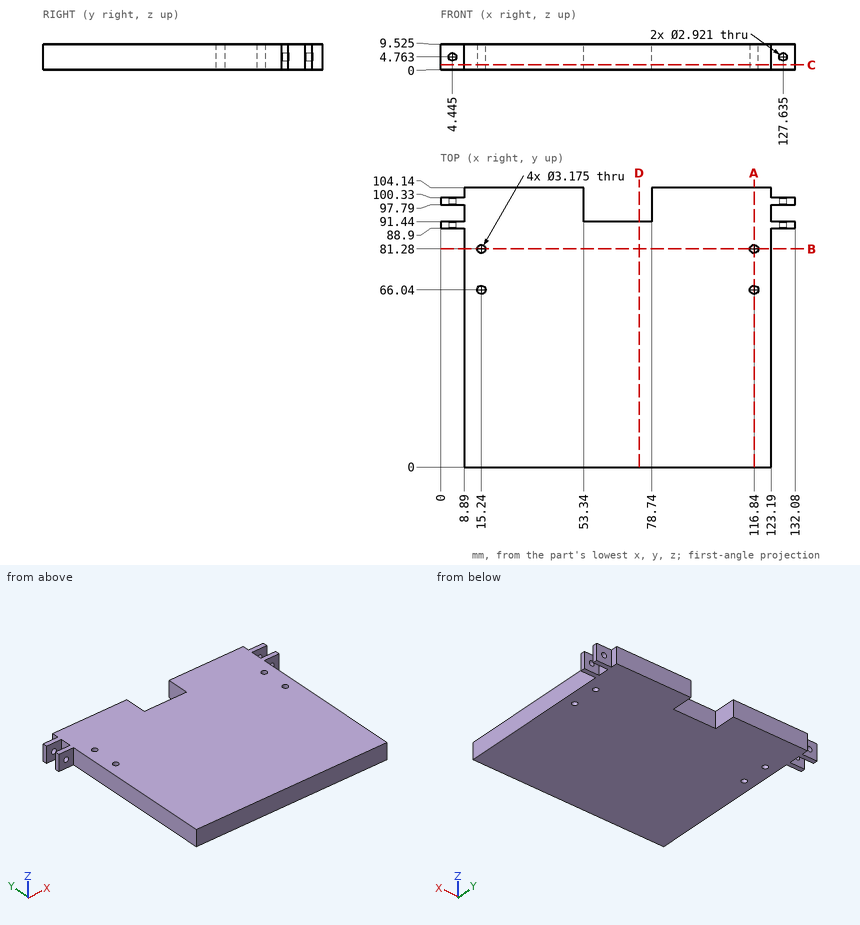
Design review of the part shown in the three views and the two pictorial views. Dimensions are in mm from the part's minimum x, y and z. Round coordinates to 2 decimals unless told otherwise and drop trailing zeros. Write each loop counter-clockwise with the first axis right and the second up, starting at its lowest first coordinate (ties: lowest second). Pieces come first, ordered by that corner, then holes. Notation, with made-up numbers: (-25.75, 83.25) - (32.25, 83.25) arc R20 ccw to (32.25, 94.25) - close; hole circle Ø3 at (63, 46.25). An arc over 180 degrees is marked (long way). Answer as CSV lines item,"result". Start each with the question number.
(1) For line 1 (X direction, y = 99.5, z = 1); line 2 (Y direction, x = 59, z = 1.25); line 3 (X direction, y = 90, z = 3.75) (1 decimal), list the stretches that pass through material, from the lowest coordinate up.
(2) Add section B-B, the plane y = 81.28. State the section outline as (x, z) points (1 decimal), plus the area to 3 significant figures.
(3) Add section C-C, the plane z = 1.75. State the section outline as (x, y) points (1 decimal).
(4) For pin 1 (4.5 mm diameter, centred on x = 4.45, z = 4.76, fed in from -Y); pin 2 (1.9 mm diameter, centred on y = 94.5, z = 3.5, fed in from +X); pin 3 (2.5 mm diameter, centred on x = 127.64, z = 4.76, fed in from +Y); pin 4 (4 mm diameter, centred on x = 15.24, y = 81.28, fed in from +Z) (1 decimal), all flat-tipped, find the tip position at first contact; note any pin that passes through.
(5) Add section D-D, the plane x = 74. State the section outline as (y, z) points (1 decimal), plus the area to 3 significant figures.
(6) Add section A-A, the plane x = 116.84. State the section outline as (y, z) points (1 decimal).
From the geometry:
1,line 1,"x = 0 to 53.34, 78.74 to 132.08"
1,line 2,"y = 0 to 91.44"
1,line 3,"x = 0 to 3.4, 5.5 to 126.6, 128.7 to 132.1"
2,outline,"(8.9, 0) - (13.7, 0) - (13.7, 9.5) - (8.9, 9.5) - close; (16.8, 0) - (115.3, 0) - (115.3, 9.5) - (16.8, 9.5) - close; (118.4, 0) - (123.2, 0) - (123.2, 9.5) - (118.4, 9.5) - close"
2,area,"1,030 mm²"
3,outline,"(0, 88.9) - (8.9, 88.9) - (8.9, 0) - (123.2, 0) - (123.2, 88.9) - (132.1, 88.9) - (132.1, 91.4) - (123.2, 91.4) - (123.2, 97.8) - (132.1, 97.8) - (132.1, 100.3) - (123.2, 100.3) - (123.2, 104.1) - (78.7, 104.1) - (78.7, 91.4) - (53.3, 91.4) - (53.3, 104.1) - (8.9, 104.1) - (8.9, 100.3) - (0, 100.3) - (0, 97.8) - (8.9, 97.8) - (8.9, 91.4) - (0, 91.4) - close; hole circle Ø3.2 at (15.2, 66); hole circle Ø3.2 at (15.2, 81.3); hole circle Ø3.2 at (116.8, 66); hole circle Ø3.2 at (116.8, 81.3)"
4,pin 1,"stops at y = 88.9"
4,pin 2,"stops at x = 123.19"
4,pin 3,"passes through"
4,pin 4,"stops at z = 9.5"
5,outline,"(0, 0) - (91.4, 0) - (91.4, 9.5) - (0, 9.5) - close"
5,area,"871 mm²"
6,outline,"(0, 0) - (64.5, 0) - (64.5, 9.5) - (0, 9.5) - close; (67.6, 0) - (79.7, 0) - (79.7, 9.5) - (67.6, 9.5) - close; (82.9, 0) - (104.1, 0) - (104.1, 9.5) - (82.9, 9.5) - close"
